Design review of the part shown in the three views and the two pictorial views. Dimensions are in mm from the part's minimum x, y and z. A direction names the side the tool comes from. Give positions to 0.01 mm unless a question says otherwise; leave off trailing zeros. Order: outer loops, then holes, each group sorted by start corner. A loop starts at its lowest first (then second) coordinate and runs counter-clockwise, first axis right, second up. Notation, with made-up numbers: M 64,79 L 117,79 A22 cw 117,93 Z; hole C 19.25,21 d9. An arc over 180 degrees is marked long. Answer as a JSON object with one key per item and string values.
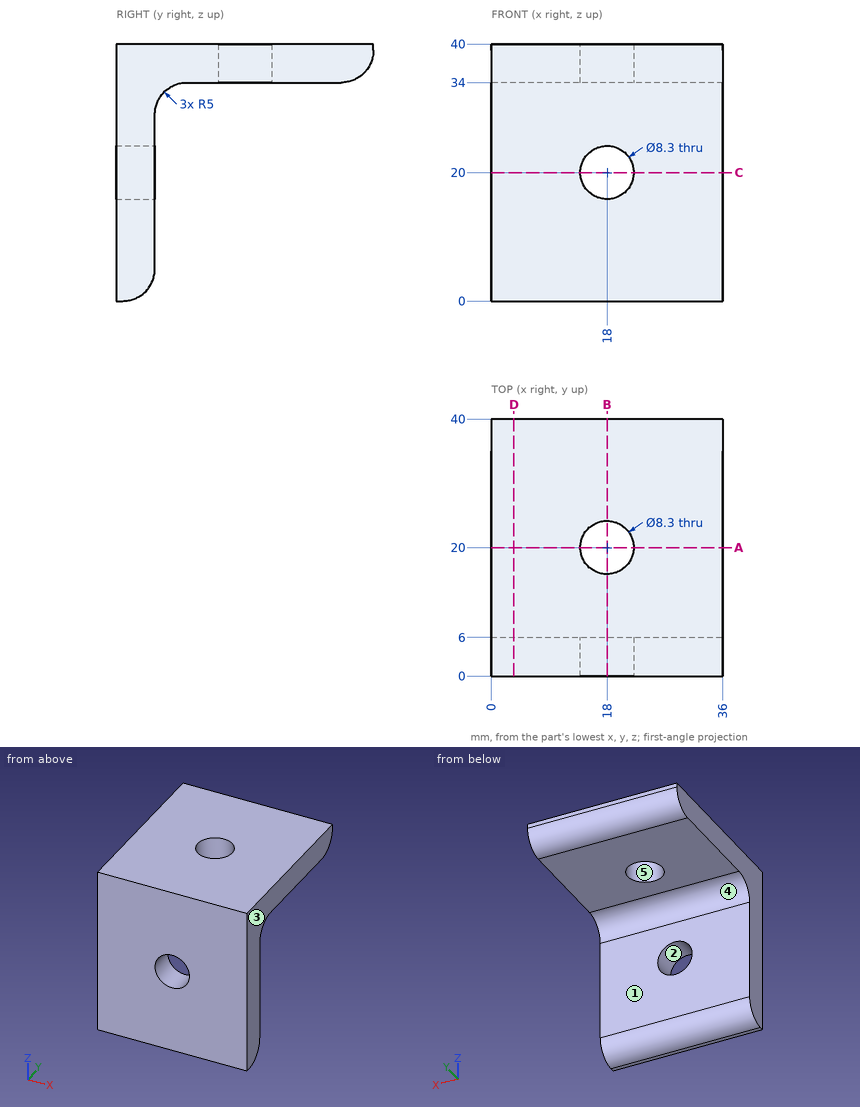
(1) Tool access review of the marked faces 1 and 2: name each direction out of +Z, -Z, +X, -X, +Y, -Y from which nothing blocks a thin tool from reaching the whole face with its end or side.
Checked values:
{"face 1": "-Z, +X, -X, +Y", "face 2": "+Y, -Y"}
(2) Draft analysis for pull direction X (two halves, no side actions). For the marked faces 3, 4 and 5, state which applies: +X half, -X half, draft (parallel to the pull), parting line (faces both ways), or undercut.
Checked values:
{"face 3": "+X half", "face 4": "draft", "face 5": "undercut"}
(3) We need section D-D (x = 3.5). Write out the cut boundary in (y, z).
Checked values:
{"outline": "M 0,0 L 1,0 A5 ccw 6,5 L 6,29 A5 cw 11,34 L 35,34 A5 ccw 40,39 L 40,40 L 0,40 Z"}
(4) We need section B-B (x = 18). Write out the cut boundary in (y, z).
Checked values:
{"outline": "M 0,0 L 1,0 A5 ccw 6,5 L 6,15.85 L 0,15.85 Z; M 0,24.15 L 6,24.15 L 6,29 A5 cw 11,34 L 15.85,34 L 15.85,40 L 0,40 Z; M 24.15,34 L 35,34 A5 ccw 40,39 L 40,40 L 24.15,40 Z"}
(5) We need section C-C (z = 20). Write out the cut boundary in (x, y), plus the area to 3 significant figures.
Checked values:
{"outline": "M 0,0 L 13.85,0 L 13.85,6 L 0,6 Z; M 22.15,0 L 36,0 L 36,6 L 22.15,6 Z", "area": "166 mm^2"}
(6) Insertion check: pin 1 (13.5 mm diameter, centred on x = 18, z = 20, fed in from +Y); pin 2 (5 mm diameter, centred on x = 18, y = 20, fed in from +Z); pin 3 (8 mm diameter, centred on x = 29, y = 14, fed in from -Z); pin 4 (10 mm diameter, centred on x = 15.5, y = 23.5, fed in from -Z). Each pin has a flat end and moves straight along its axis. Give the tip position at first contact, or say it passes through.
Checked values:
{"pin 1": "stops at y = 6", "pin 2": "passes through", "pin 3": "stops at z = 33.9", "pin 4": "stops at z = 34"}
(7) To check wall thickness, follow L1, parallel to X at y = 2.25, z = 20; L2, parallel to Z at x = 10.5, y = 16; L3, parallel to Y at x = 5, z = 8. State the ranges of each line that lie inside material, in increasing order. Write a range as from..to.
Checked values:
{"L1": "x = 0..13.85, 22.15..36", "L2": "z = 34..40", "L3": "y = 0..6"}
(8) We need section A-A (y = 20). Write out the cut boundary in (x, z).
Checked values:
{"outline": "M 0,34 L 13.85,34 L 13.85,40 L 0,40 Z; M 22.15,34 L 36,34 L 36,40 L 22.15,40 Z"}
